Input: part model. Units: mm. Frame: model coordinates. Coordinates: 2 decimals unless noted, no trailing zeros. Loops run counter-clockwise (first coordinate to the right, second up) from the corner with the lowest first, then second, coordinate; pieces in that order, holes last. Notation, with made-up numbers: (81.5, -10) - (130.5, -10) arc R26 ccw to (130.5, 28) - close; hole circle Ø5 at (-26.75, 71.25). An arc over 180 degrees is marked (long way). Use one line per item in the form item = value.
from build123d import *

# Parameters (mm, degrees)
SKETCH1_W           = 5.4
SKETCH1_H           = 5.4
SKETCH1_R           = 1.5
BOSS_EXTRUDE1_DEPTH = 2.4


with BuildPart() as part:
    # Sketch1 → Boss-Extrude1 (new body)
    with BuildSketch(Plane(origin=(0, 0, 0), x_dir=(1, 0, 0), z_dir=(0, 1, 0))):
        Rectangle(SKETCH1_W, SKETCH1_H)
        with Locations(Location((0, 0, 0), (0, 0, 270))):
            Circle(SKETCH1_R, mode=Mode.SUBTRACT)
    extrude(amount=BOSS_EXTRUDE1_DEPTH)

    # Sketch2 → Cut-Revolve1 (revolve, cut)
    with BuildSketch(Plane.XY, mode=Mode.PRIVATE) as cut_revolve1_sk:
        Polygon((-2.4, 2.4), (-4.9, 1.2), (-4.9, 2.4), align=None)
    revolve(cut_revolve1_sk.sketch.rotate(Axis((0, 2.4, 0), (0, -1, 0)), 134.999999961), axis=Axis((0, 2.4, 0), (0, -1, 0)), mode=Mode.SUBTRACT)


solid = part.part
Q1. Cut plane C-C, the plane y = 0.85. Return loops of the section in (x, z), then the cut area to 3 significant figures.
Check values:
outline = (-2.7, -2.7) - (2.7, -2.7) - (2.7, 2.7) - (-2.7, 2.7) - close; hole circle Ø3 at (0, 0)
area = 22.1 mm²
Q2. Cut plane B-B, the plane x = 0. Return loops of the section in (y, z).
Check values:
outline = (0, -2.7) - (2.26, -2.7) - (2.4, -2.4) - (2.4, -1.5) - (0, -1.5) - close; (0, 1.5) - (2.4, 1.5) - (2.4, 2.4) - (2.26, 2.7) - (0, 2.7) - close
Q3. Pull-direction query (Z, two-part tool) for faces 1 (the flat face through (0, 2.4, 2)), 2 (the flat face through (0, 1, -2.7)), 3 (the cylindrical face through (0.45, 1.18, 1.43)); classes: pulls with the +Z half, pulls with the -Z half, needs draft (parallel to the pull), parting line crosses it, or undercut.
Check values:
face_1 = needs draft
face_2 = pulls with the -Z half
face_3 = undercut
Q4. Ray query, line 1 along X through (y, z) = (1.3, 0); line 2 along X through (y, z) = (1.45, -0.7); line 3 along Z through (x, y) = (0.35, 2.05). Return the intervals inside material, ascending. Write a range as [from, to].
Check values:
line_1 = [-2.7, -1.5], [1.5, 2.7]
line_2 = [-2.7, -1.33], [1.33, 2.7]
line_3 = [-2.7, -1.46], [1.46, 2.7]
Q5. Cut plane A-A, the plane z = 0. Return loops of the section in (x, y).
Check values:
outline = (-2.7, 0) - (-1.5, 0) - (-1.5, 2.4) - (-2.4, 2.4) - (-2.7, 2.26) - close; (1.5, 0) - (2.7, 0) - (2.7, 2.26) - (2.4, 2.4) - (1.5, 2.4) - close
Q6. Cut plane D-D, the plane y = 1.95. Return loops of the section in (x, z) (1 decimal).
Check values:
outline = (-2.7, -2) arc R3.3 ccw to (-2, -2.7) - (2, -2.7) arc R3.3 ccw to (2.7, -2) - (2.7, 2) arc R3.3 ccw to (2, 2.7) - (-2, 2.7) arc R3.3 ccw to (-2.7, 2) - close; hole circle Ø3 at (0, 0)
Q7. First-contact query: P1, Ø3, axis at x = -1.5, z = 1, coming from the -Y side. Flat tip, straight axial feed; report the tip coordinate or a pass-through.
Check values:
P1 = 0
